Check sheet for the modelled part. Datum: model origin and axes. Units: mm. Give positions to 0.01 mm unless a question says otherwise; leave off trailing zeros. Order: outer loops, then holes, each group sorted by start corner. A loop starts at its lowest first (then second) coordinate and runs counter-clockwise, first axis right, second up. Notation, with made-up numbers: (74, 37.5) -> (133, 37.5) arc R28 ccw to (133, 58.5) -> close; hole circle Ø9 at (88, 48.25). An arc over 180 degrees is marked (long way). Answer in a Markdown table with one row per item. Add a question column.
(1) Cross-section at A-A (z = 8.75). Record the cut outline in (x, y).
(2) Cross-section at B-B (y = 2.4). Record the cut outline in (x, z), then the cut area to 3 significant figures.
(3) Thickness scan on L1, parallel to X at y = 0.85, z = 18.5; L2, parallel to Z at x = -3.5, y = 2.35. Record the ranges inside material, lowest first. Write a range as [from, to].
(4) Go/stop test with a flat-tipped pin: pin 1 (1.5 mm diameter, centred on x = -3.5, y = 1, fed in from -Z). Record where the tip stops, or that it passes through.
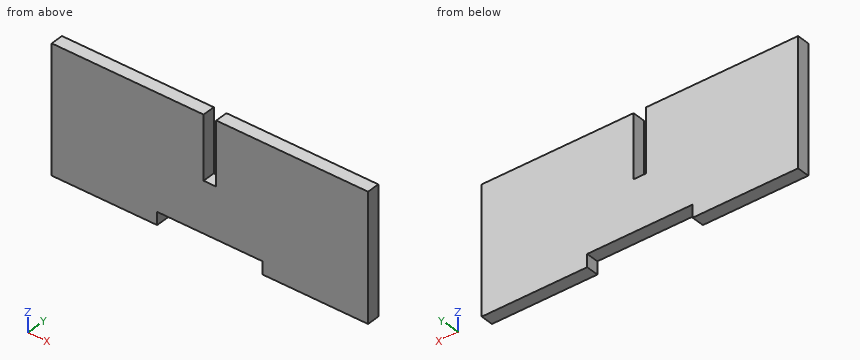
```python
from build123d import *

# Parameters (mm, degrees)
RESSALTO_EXTRUS_O1_DEPTH = 3
ESBO_O2_W                = 25
ESBO_O2_H                = 12.767391237
CORTE_EXTRUS_O1_DEPTH    = 3


with BuildPart() as part:
    # Esboço1 → Ressalto-extrusão1 (new body)
    with BuildSketch(Plane(origin=(0, 0, 0), x_dir=(1, 0, 0), z_dir=(0, 1, 0))):
        Polygon((36, 7.331730769), (-39, 7.331730769), (-39, -22.668269231), (-3, -22.668269231), (-3, -7.668269231), (0, -7.668269231), (0, -22.668269231), (36, -22.668269231), align=None)
    extrude(amount=RESSALTO_EXTRUS_O1_DEPTH)

    # Esboço2 → Corte-extrusão1 (cut)
    with BuildSketch(Plane(origin=(0, 0, -7.331730769), x_dir=(-1, 0, 0), z_dir=(0, 0, -1))):
        with Locations((1.5, 0.308837842)):
            Rectangle(ESBO_O2_W, ESBO_O2_H)
    extrude(amount=-CORTE_EXTRUS_O1_DEPTH, mode=Mode.SUBTRACT)


solid = part.part
```
Answer below:
| question | item | result |
|---|---|---|
| 1 | outline | (-39, 0) -> (-3, 0) -> (-3, 3) -> (-39, 3) -> close; (0, 0) -> (36, 0) -> (36, 3) -> (0, 3) -> close |
| 2 | outline | (-39, -7.33) -> (-14, -7.33) -> (-14, -4.33) -> (11, -4.33) -> (11, -7.33) -> (36, -7.33) -> (36, 22.67) -> (0, 22.67) -> (0, 7.67) -> (-3, 7.67) -> (-3, 22.67) -> (-39, 22.67) -> close |
| 2 | area | 2,130 mm² |
| 3 | L1 | x = [-39, -3], [0, 36] |
| 3 | L2 | z = [-4.33, 22.67] |
| 4 | pin 1 | stops at z = -4.33 |
